Input: dimensioned drawing with shaded views. Units: mm. Origin: part minimum x, y, z. Give positions to 0.01 mm unless a question says otherwise; leave off trailing zeros. Write each loop counter-clockwise with the first axis right and the second up, starting at its lowest first coordinate (ties: lowest second). Pieces come first, ordered by that corner, then holes. Notation, with made-up numbers: (-32.75, -38) -> (-20.75, -38) arc R23 cw to (-20.75, 0) -> close; hole circle Ø8 at (22, -34). An arc over 180 degrees is marked (long way). Return JSON: item names as keys, results as strings. Group by question number.
Item 1: Mould query, pull axis Z, two halves, no side actions, for the marked faces 1, 2 and 3. Classes: released by +Z, released by -Z, zero draft, split by the parting line, or undercut.
Item 2: Section B-B, the plane x = 75. Return loops of the section in (y, z).
Item 3: Line query: line 1 (Z direction, x = 16.5, y = 80); line 2 (Z direction, x = 63, y = 26.5); line 3 (Y direction, x = 59.5, z = 54.5). Output: solid intervals per line, ascending. Write a range as [from, to].
Item 4: Section A-A, the plane z = 39.5. Return loops of the section in (x, y), then the cut area to 3 significant figures.
Item 5: Pin query (flat end, axial travel): P1, Ø9, axis at x = 39.5, y = 71, coming from the -Z side; P2, Ø5, axis at x = 106, y = 42, coming from the -Z side; P3, Ø19, axis at x = 82.5, z = 47.5, coming from the +Y side. Return the tip coordinate at first contact, or that it passes through.
Item 6: Section C-C, the plane y = 50. Return loops of the section in (x, z), then the cut area to 3 significant figures.
Item 7: Section D-D, the plane z = 140. Return loops of the section in (x, y).
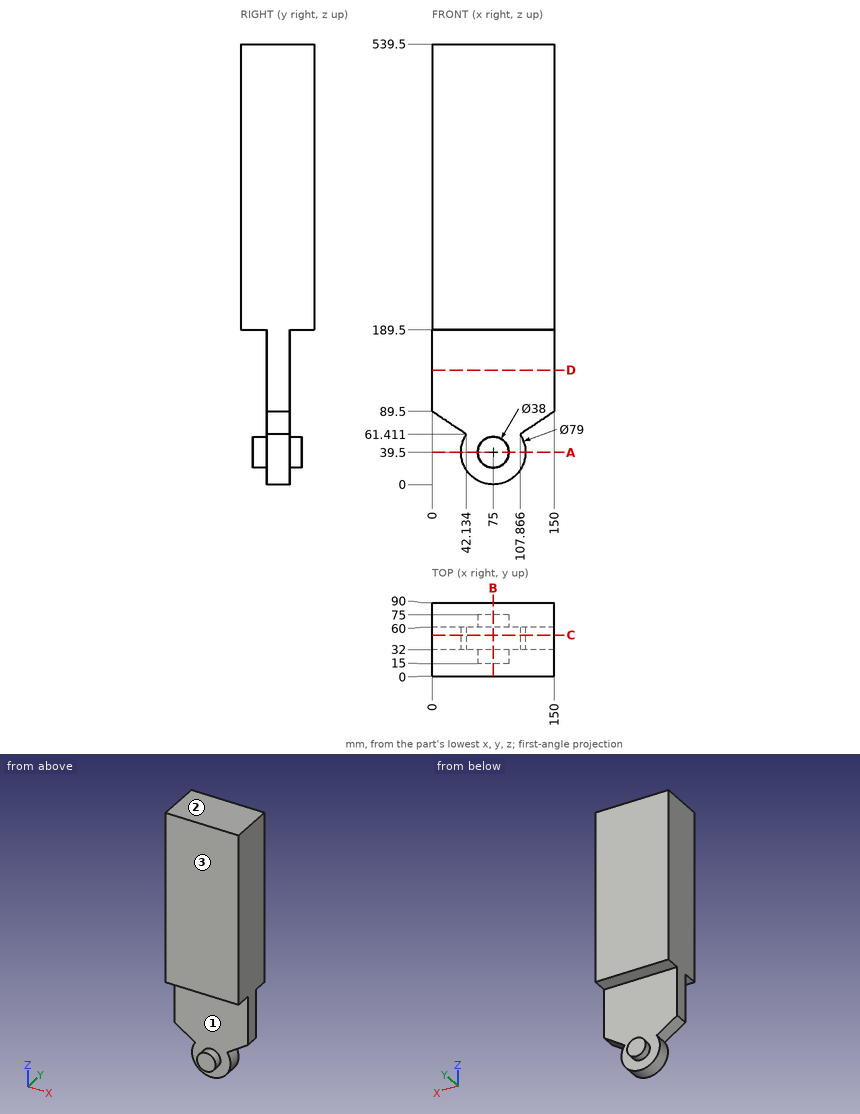
Answer below:
{
 "1": {"face 1": "undercut", "face 2": "released by +Z", "face 3": "zero draft"},
 "2": {"outline": "(0, 189.5) -> (32, 189.5) -> (32, 58.5) -> (15, 58.5) -> (15, 20.5) -> (32, 20.5) -> (32, 0) -> (60, 0) -> (60, 20.5) -> (75, 20.5) -> (75, 58.5) -> (60, 58.5) -> (60, 189.5) -> (90, 189.5) -> (90, 539.5) -> (0, 539.5) -> close"},
 "3": {"line 1": "z = [189.5, 539.5]", "line 2": "z = [24.77, 54.23], [189.5, 539.5]", "line 3": "y = [32, 60]"},
 "4": {"outline": "(35.5, 32) -> (56, 32) -> (56, 15) -> (94, 15) -> (94, 32) -> (114.5, 32) -> (114.5, 60) -> (94, 60) -> (94, 75) -> (56, 75) -> (56, 60) -> (35.5, 60) -> close", "area": "3,430 mm2"},
 "5": {"P1": "stops at z = 189.5", "P2": "stops at z = 12.15", "P3": "stops at y = 75"},
 "6": {"outline": "(0, 89.5) -> (42.13, 61.41) arc R39.5 ccw (long way) to (107.87, 61.41) -> (150, 89.5) -> (150, 539.5) -> (0, 539.5) -> close", "area": "74,600 mm2"},
 "7": {"outline": "(0, 32) -> (150, 32) -> (150, 60) -> (0, 60) -> close"}
}
